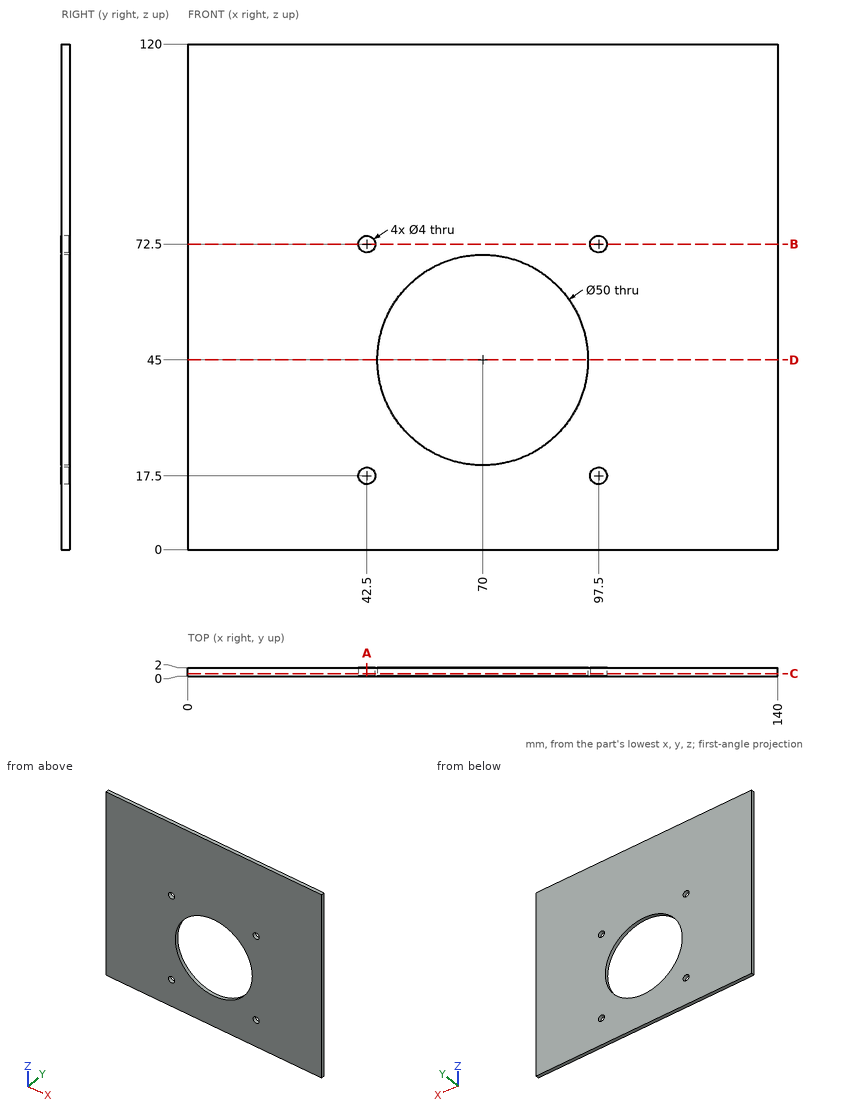
For this review, use the dimensioned drawing (mm, ordinates from the lowest corner) and the shaded views. Give positions to 0.01 mm unless a question says otherwise; leave off trailing zeros. Order: outer loops, then holes, each group sorted by start corner. A loop starts at its lowest first (then second) coordinate and runs counter-clockwise, first axis right, second up. Notation, with made-up numbers: (62.25, 65.25) - (119.25, 65.25) arc R10 ccw to (119.25, 74.25) - close; hole circle Ø3 at (16, -20.5). An arc over 180 degrees is marked (long way). Use CSV: the item, a comma, the result in double quotes. Start each with the question number.
Q1. Take a section at D-D (z = 45). State the section outline as (x, y) points.
Q2. Take a section at A-A (x = 42.5). State the section outline as (y, z) points, and give its area (3 significant figures).
Q3. Take a section at C-C (y = 0.55). State the section outline as (x, z) points.
Q4. For line 1 (X direction, y = 0.9, z = 72.5); line 2 (Z direction, x = 97.5, y = 1.3); line 3 (X direction, y = 1.5, z = 45), list the stretches that pass through material, from the lowest coordinate up.
Q5. Take a section at B-B (z = 72.5). State the section outline as (x, y) points, and give its area (3 significant figures).
Calculated:
1,outline,"(0, 0) - (45, 0) - (45, 2) - (0, 2) - close; (95, 0) - (140, 0) - (140, 2) - (95, 2) - close"
2,outline,"(0, 0) - (2, 0) - (2, 15.5) - (0, 15.5) - close; (0, 19.5) - (2, 19.5) - (2, 70.5) - (0, 70.5) - close; (0, 74.5) - (2, 74.5) - (2, 120) - (0, 120) - close"
2,area,"224 mm²"
3,outline,"(0, 0) - (140, 0) - (140, 120) - (0, 120) - close; hole circle Ø4 at (42.5, 17.5); hole circle Ø4 at (42.5, 72.5); hole circle Ø50 at (70, 45); hole circle Ø4 at (97.5, 17.5); hole circle Ø4 at (97.5, 72.5)"
4,line 1,"x = 0 to 40.5, 44.5 to 95.5, 99.5 to 140"
4,line 2,"z = 0 to 15.5, 19.5 to 70.5, 74.5 to 120"
4,line 3,"x = 0 to 45, 95 to 140"
5,outline,"(0, 0) - (40.5, 0) - (40.5, 2) - (0, 2) - close; (44.5, 0) - (95.5, 0) - (95.5, 2) - (44.5, 2) - close; (99.5, 0) - (140, 0) - (140, 2) - (99.5, 2) - close"
5,area,"264 mm²"
